Print and shaded views of the part. All mm, measured from the part's lowest x, y and z. A direction names the side the tool comes from. Round coordinates to 2 decimals unless told otherwise and drop trailing zeros. Order: outer loops, then holes, each group sorted by start corner. A loop starts at its lowest first (then second) coordinate and runs counter-clockwise, first axis right, second up. Notation, with made-up numbers: (75.25, -28) - (122.25, -28) arc R20 ccw to (122.25, -4) - close; hole circle Ø6 at (38, 24.5). An arc over 180 degrees is marked (long way). Write item = value, one per line.
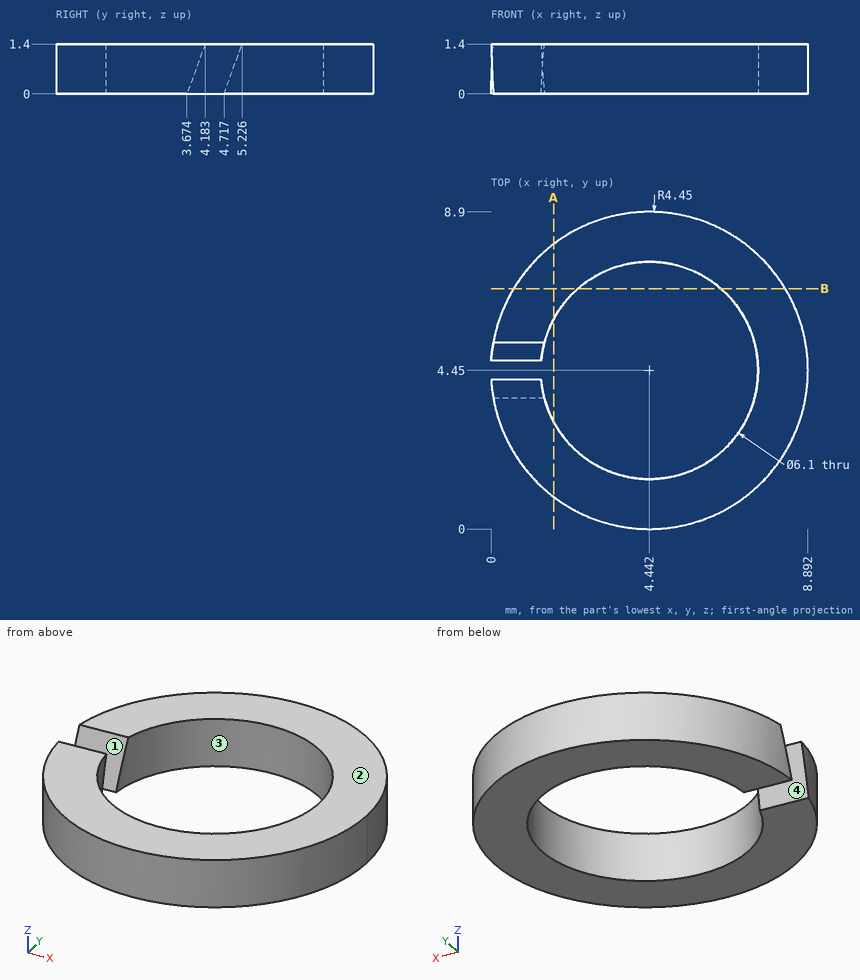
(1) Tool access for the marked faces 1 and 2: list every direction of +Z, -Z, +X, -X, +Y, -Y with a clear straight run to the whole face (end or side of a thin tool).
Solved:
face_1 = +Z, -X
face_2 = +Z, +X, -X, +Y, -Y
(2) Probe line 1 along X through (y, z) = (4.45, 0.6); line 2 along Y through (x, z) = (4, 1.25); line 3 along X through (y, z) = (6.5, 0.7) (1 decimal). List the from-to ranges inside material, lowest first.
Solved:
line_1 = 7.49 to 8.89
line_2 = 0.02 to 1.43, 7.47 to 8.88
line_3 = 0.5 to 2.2, 6.7 to 8.4
(3) Pull direction X, two halves, no side cores. Call the marked faces 3 and 4: released by +X, released by -X, zero draft, split by the parting line, or undercut.
Solved:
face_3 = undercut
face_4 = zero draft
(4) Band-saw the part on B-B on y = 6.75. List the corners of the cut face in (x, z) (1 decimal).
Solved:
outline = (0.6, 0) - (2.4, 0) - (2.4, 1.4) - (0.6, 1.4) - close; (6.4, 0) - (8.3, 0) - (8.3, 1.4) - (6.4, 1.4) - close
(5) Band-saw the part on A-A on x = 1.75. List the corners of the cut face in (y, z).
Solved:
outline = (0.91, 0) - (3.02, 0) - (3.02, 1.4) - (0.91, 1.4) - close; (5.88, 0) - (7.99, 0) - (7.99, 1.4) - (5.88, 1.4) - close
